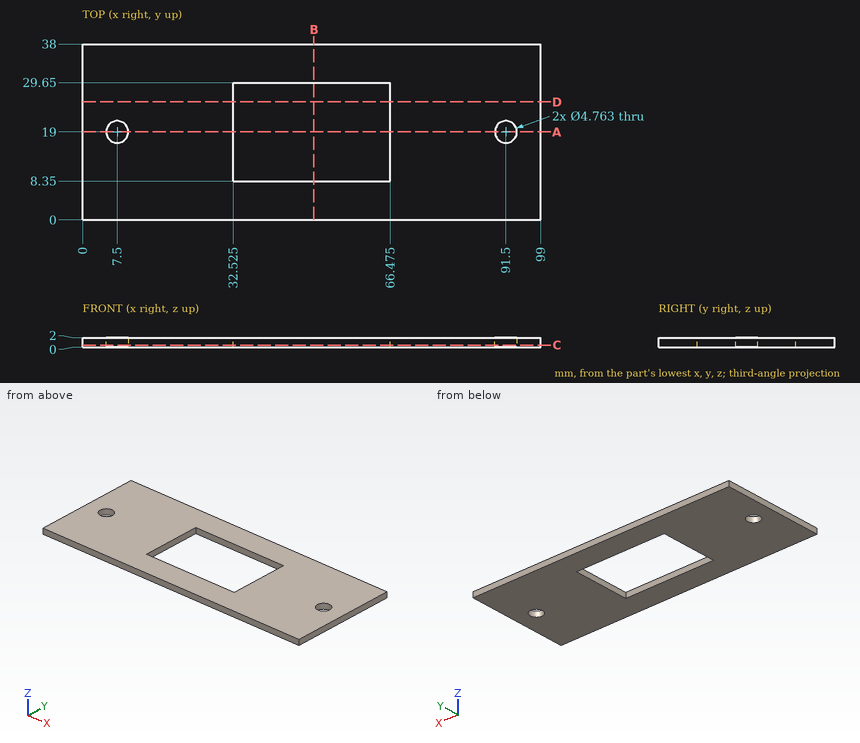
Answer from the drawing. Dimensions are ordinates in mm from the lowest x, y and z of the part. Round coordinates to 2 decimals unless told otherwise and drop trailing zeros. Loops run counter-clockwise (first coordinate to the right, second up) from the corner with the lowest first, then second, coordinate; pieces in that order, holes last.
(1) Find the intervals of material crossed by L1, parallel to Y at x = 46, z = 1; L2, parallel to X at y = 22, z = 0.5 (1 decimal); L3, parallel to Y at x = 91.5, z = 0.95, in increasing order.
Computed values:
L1: y = 0 to 8.35, 29.65 to 38
L2: x = 0 to 32.5, 66.5 to 99
L3: y = 0 to 16.62, 21.38 to 38
(2) The part is cut by section D-D, the plane y = 25.5. Give the vertices of the cut face in (x, z) (1 decimal), and give its area (3 significant figures).
Computed values:
outline: (0, 0) - (32.5, 0) - (32.5, 2) - (0, 2) - close; (66.5, 0) - (99, 0) - (99, 2) - (66.5, 2) - close
area: 130 mm2
(3) The part is cut by section A-A, the plane y = 19. Give the vertices of the cut face in (x, z) (1 decimal).
Computed values:
outline: (0, 0) - (5.1, 0) - (5.1, 2) - (0, 2) - close; (9.9, 0) - (32.5, 0) - (32.5, 2) - (9.9, 2) - close; (66.5, 0) - (89.1, 0) - (89.1, 2) - (66.5, 2) - close; (93.9, 0) - (99, 0) - (99, 2) - (93.9, 2) - close
(4) The part is cut by section C-C, the plane z = 0.45. Give the number of separate pieces and of enclosed holes in the cut face, and give its area (3 significant figures).
Computed values:
separate pieces: 1
enclosed holes: 3
area: 3,000 mm2
(5) Each of these flat-tipped pins is pushed along its axis until it touches: P1, Ø4, axis at x = 28, y = 25, coming from the -Z side; P2, Ø4.5, axis at x = 91.5, y = 19, coming from the -Z side. Where does it stop, or does it pass through?
Computed values:
P1: stops at z = 0
P2: passes through
(6) The part is cut by section B-B, the plane x = 50. Give the vertices of the cut face in (y, z).
Computed values:
outline: (0, 0) - (8.35, 0) - (8.35, 2) - (0, 2) - close; (29.65, 0) - (38, 0) - (38, 2) - (29.65, 2) - close
